Verification items for the finished model (mm, model axes). Face numbers are marked on the shaded views. A direction names the side the tool comes from. Round coordinates to 2 decimals unless told otherwise and drop trailing zeros. Order: outer loops, then holes, each group sorted by start corner. A loop starts at its lowest first (then second) coordinate and runs counter-clockwise, first axis right, second up. Notation, with made-up numbers: (24, 32) -> (66, 32) arc R16 cw to (66, 43) -> close; hole circle Ø2 at (7, 58). An arc over 180 degrees is marked (long way). Write item = value, one per line. Start each with the question number.
from build123d import *

# Parameters (mm, degrees)
SKETCH2_W                 = 34.29
SKETCH2_H                 = 21.59
SKETCH2_R                 = 1.27
PCB_DEPTH                 = 1.6
FILLET1_R                 = 1.27
SKETCH3_W                 = 6
SKETCH3_H                 = 5
CONTROL_CONNECTOR_DEPTH   = 5.6
SKETCH3_3_W               = 12
SKETCH3_3_H               = 6
ELECTRODE_CONNECTOR_DEPTH = 4.4
SKETCH3_4_W               = 7.3
SKETCH3_4_H               = 10.795
SKETCH3_4_H_2             = 3.905
RELAY_DEPTH               = 9.9


with BuildPart() as part:
    # Sketch2 → PCB (new body)
    with BuildSketch(Plane(origin=(0, 0, 0), x_dir=(1, 0, 0), z_dir=(0, 1, 0))):
        Rectangle(SKETCH2_W, SKETCH2_H)
        with Locations(Location((-14.605, 8.255, 0), (0, 0, 270))):
            Circle(SKETCH2_R, mode=Mode.SUBTRACT)
        with Locations(Location((14.605, 8.255, 0), (0, 0, 90))):
            Circle(SKETCH2_R, mode=Mode.SUBTRACT)
        with Locations(Location((14.605, -8.255, 0), (0, 0, 270))):
            Circle(SKETCH2_R, mode=Mode.SUBTRACT)
        with Locations(Location((-14.605, -8.255, 0), (0, 0, 90))):
            Circle(SKETCH2_R, mode=Mode.SUBTRACT)
    extrude(amount=PCB_DEPTH)

    # Fillet1
    fillet1_edges = [part.edges().sort_by_distance(p)[0] for p in [
        (17.145, 0.8, 10.795),
        (-17.145, 0.8, 10.795),
        (-17.145, 0.8, -10.795),
        (17.145, 0.8, -10.795),
    ]]
    fillet(fillet1_edges, radius=FILLET1_R)

    # Sketch3 → Control_connector (add)
    with BuildSketch(Plane(origin=(0, 1.6, 0), x_dir=(1, 0, 0), z_dir=(0, 1, 0))):
        with Locations((-14.145, 2.5)):
            Rectangle(SKETCH3_W, SKETCH3_H)
        with Locations((-14.145, -2.5)):
            Rectangle(SKETCH3_W, SKETCH3_H)
    extrude(amount=CONTROL_CONNECTOR_DEPTH)

    # Sketch3_3 → Electrode_connector (add)
    with BuildSketch(Plane(origin=(0, 1.6, 0), x_dir=(1, 0, 0), z_dir=(0, 1, 0))):
        with Locations((11.145, 3)):
            Rectangle(SKETCH3_3_W, SKETCH3_3_H)
        with Locations((11.145, -3)):
            Rectangle(SKETCH3_3_W, SKETCH3_3_H)
    extrude(amount=ELECTRODE_CONNECTOR_DEPTH)

    # Sketch3_4 → Relay (add)
    with BuildSketch(Plane(origin=(0, 1.6, 0), x_dir=(1, 0, 0), z_dir=(0, 1, 0))):
        with Locations((-3.195, 5.3975)):
            Rectangle(SKETCH3_4_W, SKETCH3_4_H)
        with Locations((-3.195, -1.9525)):
            Rectangle(SKETCH3_4_W, SKETCH3_4_H_2)
    extrude(amount=RELAY_DEPTH)


solid = part.part
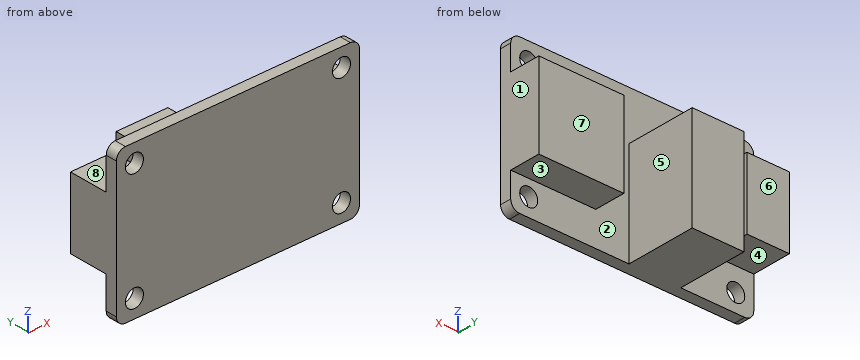
(1) Scan lines: line 1 along X through (y, z) = (3.25, 3.75) (3 decimals); line 2 along X through (y, z) = (6.25, -1) (3 decimals); line 3 along Z through (x, y) = (13.5, 1) (3 decimals). Record each from-to range of solid material in increasing order. Write a range as from..to.
(2) Set-up check for the marked faces 4, 5, 6, 7 and 8: record each of +Z, -Z, +X, -X, +Y, -Y from which the full face is reachable in a straight line by a thin tool's end or side.
(3) Draft check along X on the marked faces 1, 2 and 3. Enter one of: +X half, -X half, draft (parallel to the pull), parting line (faces both ways), or undercut.
(4) Cross-section at A-A (y = 3.25). Enter the section's corners in (x, z) (3 decimals).
(5) Cross-section at B-B (z = 0.25). Enter the section's corners in (x, y) (3 decimals), and give its area (3 significant figures).
(6) Cross-section at C-C (x = 6.5). Enter the section's corners in (y, z) (3 decimals).
(7) Depth check by flat-ended pin: pin 1 (1.7 mm diameter, centred on x = -13, y = 4, fed in from -Z); pin 2 (5 mm diameter, centred on y = 8.5, z = -4.5, fed in from -X) (3 decimals); pin 3 (6.5 mm diameter, centred on x = 5, z = -1.5, fed in from +Y); pin 4 (4 mm diameter, centred on x = 14.605, z = -8.255, fed in from +Y). Enter the tip coordinate at first touch or a pass-through.
(8) Cross-section at D-D (y = 8.25). Enter the section's corners in (x, z) (3 decimals), and give its area (3 significant figures).
Outcome:
q1.line_1 = -17.145..-11.145, -6.845..0.455, 5.145..17.145
q1.line_2 = -17.145..-11.145, -6.845..0.455
q1.line_3 = -10.795..-8.881, -7.629..7.629, 8.881..10.795
q2.face_4 = -Z, -X, +Y
q2.face_5 = +Z, -Z, +Y
q2.face_6 = +Z, -Z, -X, +Y
q2.face_7 = +Z, -Z, +X, +Y
q2.face_8 = +Z, -X, +Y
q3.face_1 = +X half
q3.face_2 = undercut
q3.face_3 = draft
q4.outline = (-17.145, -5) -> (-11.145, -5) -> (-11.145, 5) -> (-17.145, 5) -> close; (-6.845, -10.795) -> (0.455, -10.795) -> (0.455, 3.905) -> (-6.845, 3.905) -> close; (5.145, -6) -> (17.145, -6) -> (17.145, 6) -> (5.145, 6) -> close
q5.outline = (-17.145, 0) -> (17.145, 0) -> (17.145, 6) -> (5.145, 6) -> (5.145, 1.6) -> (0.455, 1.6) -> (0.455, 11.5) -> (-6.845, 11.5) -> (-6.845, 1.6) -> (-11.145, 1.6) -> (-11.145, 7.2) -> (-17.145, 7.2) -> close
q5.area = 214 mm^2
q6.outline = (0, -10.795) -> (1.6, -10.795) -> (1.6, -6) -> (6, -6) -> (6, 6) -> (1.6, 6) -> (1.6, 10.795) -> (0, 10.795) -> close
q7.pin_1 = -5
q7.pin_2 = -17.145
q7.pin_3 = 6
q7.pin_4 = 1.6
q8.outline = (-6.845, -10.795) -> (0.455, -10.795) -> (0.455, 3.905) -> (-6.845, 3.905) -> close
q8.area = 107 mm^2
